Design review of the part built by this model. Coordinates are the model's own, in mm. Face numbers are marked on the shaded views. A direction names the side the tool comes from. Give positions to 0.01 mm unless a question says otherwise; leave off trailing zeros. Write each loop counter-clockwise with the first axis right and the second up, starting at its lowest first coordinate (ties: lowest second). Pieces come first, ordered by that corner, then holes. Notation, with made-up numbers: (36, 89.5) - (70, 89.5) arc R21 cw to (70, 105.5) - close; hole circle Ø8 at (7, 58). An arc over 180 degrees is marked (long way). Write each question's results on one line, items separated by ' | '. Start each with the question number.
from build123d import *

# Parameters (mm, degrees)
SCHIZZO1_W                   = 10
SCHIZZO1_H                   = 10
ESTRUSIONE_ESTRUSIONE1_DEPTH = 10
FORO_FILETTATO_M3X0_5_1_D    = 2.5
FORO_FILETTATO_M3X0_5_2_D    = 2.5
FORO_FILETTATO_M3X0_5_3_D    = 2.5
SCHIZZO8_R                   = 3
TAGLIO_ESTRUSIONE1_DEPTH     = 8
SCHIZZO9_R                   = 3
TAGLIO_ESTRUSIONE2_DEPTH     = 8
SCHIZZO10_R                  = 3
TAGLIO_ESTRUSIONE3_DEPTH     = 8


with BuildPart() as part:
    # Schizzo1 → Estrusione-Estrusione1 (new body)
    with BuildSketch(Plane.XY):
        Rectangle(SCHIZZO1_W, SCHIZZO1_H)
    extrude(amount=ESTRUSIONE_ESTRUSIONE1_DEPTH)

    # Foro filettato M3x0.5-1 (through all)
    with Locations(Plane.XY.offset(10)):
        with Locations((0, 0)):
            Hole(FORO_FILETTATO_M3X0_5_1_D / 2)

    # Foro filettato M3x0.5-2 (through all)
    with Locations(Plane(origin=(5, 0, 0), x_dir=(0, 0, -1), z_dir=(1, 0, 0))):
        with Locations((-5, 0)):
            Hole(FORO_FILETTATO_M3X0_5_2_D / 2)

    # Foro filettato M3x0.5-3 (through all)
    with Locations(Plane(origin=(0, -5, 0), x_dir=(-1, 0, 0), z_dir=(0, -1, 0))):
        with Locations((0, -5)):
            Hole(FORO_FILETTATO_M3X0_5_3_D / 2)

    # Schizzo8 → Taglio-Estrusione1 (cut)
    with BuildSketch(Plane.XY.offset(10)):
        Circle(SCHIZZO8_R)
    extrude(amount=-TAGLIO_ESTRUSIONE1_DEPTH, mode=Mode.SUBTRACT)

    # Schizzo9 → Taglio-Estrusione2 (cut)
    with BuildSketch(Plane(origin=(5, 0, 0), x_dir=(0, 0, -1), z_dir=(1, 0, 0))):
        with Locations((-5, 0)):
            Circle(SCHIZZO9_R)
    extrude(amount=-TAGLIO_ESTRUSIONE2_DEPTH, mode=Mode.SUBTRACT)

    # Schizzo10 → Taglio-Estrusione3 (cut)
    with BuildSketch(Plane(origin=(0, 5, 0), x_dir=(1, 0, 0), z_dir=(0, 1, 0))):
        with Locations((0, -5)):
            Circle(SCHIZZO10_R)
    extrude(amount=-TAGLIO_ESTRUSIONE3_DEPTH, mode=Mode.SUBTRACT)


solid = part.part
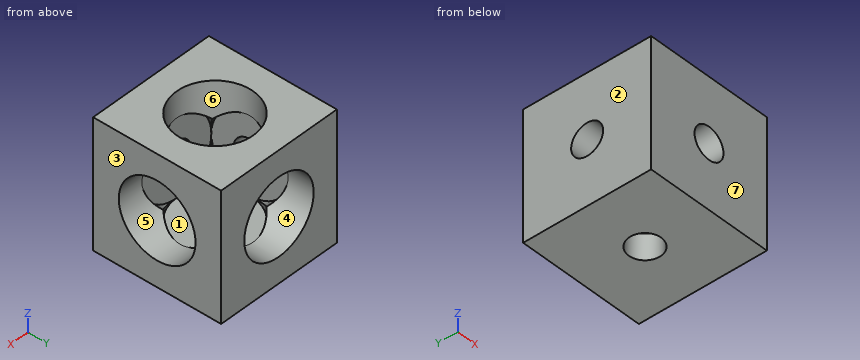
Q1. Add section A-A on x = -3.25. State the section outline as (y, z) points, plus the area to 3 significant figures.
Q2. Add section D-D on x = -0.5. State the section outline as (y, z) points, plus the area to 3 significant figures.
Q3. Add section B-B on z = 6.75. State the section outline as (x, y) points, plus the area to 3 significant figures.
Q4. For line 1 along Y through (x, z) = (0, 8.6); line 2 along Z through (x, y) = (0, -4.45); line 3 along Y through (x, z) = (0, 1.3), list the stretches that pass through material, from the lowest coordinate up. Write a range as [from, to].
Q5. Insertion check: P1, Ø5, axis at x = 0, z = 5, coming from the +Y side; P2, Ø2, axis at x = 0, y = 0, coming from the -Z side. Each pin has a flat end and moves straight along its axis. Give the tip position at first contact, or say it passes through.
Q6. The part is to be moulded in two halves that separate along X. For the marked faces 1, 2 and 3, say which applies: +X half, -X half, draft (parallel to the pull), parting line (faces both ways), or undercut.
Q7. Machinability: for the marked faces 4, 5, 6 and 7, which of the approach directions +Z, -Z, +X, -X, +Y, -Y give a long, thin tool a straight path to every point of the face, cutting with its end or side? Answer none if there is none.
Result:
1) outline: (-5, 0) - (5, 0) - (5, 10) - (-5, 10) - close; hole circle Ø2.5 at (0, 5) | area: 95.1 mm²
2) outline: (-5, 0) - (-1.15, 0) - (-1.15, 2) - (-2.96, 2) - (-2.96, 2.04) - (-3, 2.04) - (-3, 3.85) - (-5, 3.85) - close; (-5, 6.15) - (-3, 6.15) - (-3, 7.96) - (-2.96, 7.96) - (-2.96, 10) - (-5, 10) - close; (1.15, 0) - (5, 0) - (5, 2.04) - (2.96, 2.04) - (2.96, 2) - (1.15, 2) - close; (2.96, 7.96) - (5, 7.96) - (5, 10) - (2.96, 10) - close | area: 31.2 mm²
3) outline: (-5, -5) - (5, -5) - (5, -2.44) - (2.44, -2.44) - (2.44, -3) - (-2.44, -3) - (-2.44, -2.44) - (-3, -2.44) - (-3, 2.44) - (-2.44, 2.44) - (-2.44, 5) - (-5, 5) - close; (2.44, 2.44) - (5, 2.44) - (5, 5) - (2.44, 5) - close | area: 45.8 mm²
4) line 1: y = [-5, -3], [3, 5] | line 2: z = [0, 3.75], [6.25, 10] | line 3: y = [-5, -1.25], [1.25, 5]
5) P1: stops at y = -3 | P2: passes through
6) face 1: undercut | face 2: -X half | face 3: +X half
7) face 4: +Y | face 5: +X | face 6: +Z | face 7: +Z, -Z, +X, -X, -Y
